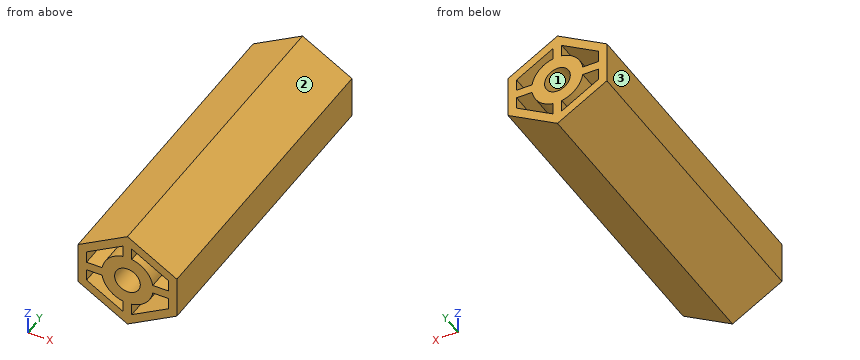
from build123d import *

# Parameters (mm, degrees)
SKETCH1_R           = 3.25
BOSS_EXTRUDE2_DEPTH = 80


with BuildPart() as part:
    # Sketch1 → Boss-Extrude2 (new body)
    with BuildSketch(Plane(origin=(0, 0, 0), x_dir=(1, 0, 0), z_dir=(0, 1, 0))):
        Polygon((-12.5, 5.283121635), (-12.5, -5.283121635), (0, -12.5), (12.5, -5.283121635), (12.5, 5.283121635), (0, 12.5), align=None)
        Circle(SKETCH1_R, mode=Mode.SUBTRACT)
        with BuildLine():
            Line((-1.08, 9.382308546), (-1.08, 6.409648976))
            ThreePointArc((-1.08, 6.409648976), (-4.596194078, 4.596194078), (-6.409648976, 1.08))
            Line((-6.409648976, 1.08), (-10.34, 1.08))
            Line((-10.34, 1.08), (-10.34, 4.036045054))
            Line((-10.34, 4.036045054), (-1.08, 9.382308546))
        make_face(mode=Mode.SUBTRACT)
        with BuildLine():
            Line((1.08, 9.382308546), (1.08, 6.409648976))
            ThreePointArc((1.08, 6.409648976), (4.596194078, 4.596194078), (6.409648976, 1.08))
            Line((6.409648976, 1.08), (10.34, 1.08))
            Line((10.34, 1.08), (10.34, 4.036045054))
            Line((10.34, 4.036045054), (1.08, 9.382308546))
        make_face(mode=Mode.SUBTRACT)
        with BuildLine():
            Line((-10.34, -1.08), (-6.409648976, -1.08))
            ThreePointArc((-6.409648976, -1.08), (-4.596194078, -4.596194078), (-1.08, -6.409648976))
            Line((-1.08, -6.409648976), (-1.08, -9.382308546))
            Line((-1.08, -9.382308546), (-10.34, -4.036045054))
            Line((-10.34, -4.036045054), (-10.34, -1.08))
        make_face(mode=Mode.SUBTRACT)
        with BuildLine():
            Line((1.08, -6.409648976), (1.08, -9.382308546))
            Line((1.08, -9.382308546), (10.34, -4.036045054))
            Line((10.34, -4.036045054), (10.34, -1.08))
            Line((10.34, -1.08), (6.409648976, -1.08))
            ThreePointArc((6.409648976, -1.08), (4.596194078, -4.596194078), (1.08, -6.409648976))
        make_face(mode=Mode.SUBTRACT)
    extrude(amount=BOSS_EXTRUDE2_DEPTH)


solid = part.part
Verification items for the finished model (mm, model axes). Face numbers are marked on the shaded views. Coordinates: 2 decimals unless noted, no trailing zeros. Loops run counter-clockwise (first coordinate to the right, second up) from the corner with the lowest first, then second, coordinate; pieces in that order, holes last. Notation, with made-up numbers: M -33.75,-37 L 18.25,-37 A21 cw 18.25,-30 Z; hole C -28,-6.5 d11. An arc over 180 degrees is marked long. One line per item, written item: value.
1. Section check B-B on x = -4. Record the cut outline in (y, z).
Answers follow:
outline: M 0,-10.19 L 80,-10.19 L 80,-7.7 L 0,-7.7 Z; M 0,-5.12 L 80,-5.12 L 80,5.12 L 0,5.12 Z; M 0,7.7 L 80,7.7 L 80,10.19 L 0,10.19 Z
2. Section check C-C on y = 24.5. Record the cut outline in (x, z).
Answers follow:
outline: M -12.5,-5.28 L 0,-12.5 L 12.5,-5.28 L 12.5,5.28 L 0,12.5 L -12.5,5.28 Z; hole M -10.34,-4.04 L -1.08,-9.38 L -1.08,-6.41 A6.5 cw -6.41,-1.08 L -10.34,-1.08 Z; hole M -10.34,1.08 L -6.41,1.08 A6.5 cw -1.08,6.41 L -1.08,9.38 L -10.34,4.04 Z; hole C 0,0 d6.5; hole M 1.08,-9.38 L 10.34,-4.04 L 10.34,-1.08 L 6.41,-1.08 A6.5 cw 1.08,-6.41 Z; hole M 1.08,6.41 A6.5 cw 6.41,1.08 L 10.34,1.08 L 10.34,4.04 L 1.08,9.38 Z
3. Section check D-D on z = -7.5. Record the cut outline in (x, y).
Answers follow:
outline: M -8.66,0 L -4.34,0 L -4.34,80 L -8.66,80 Z; M -1.08,0 L 1.08,0 L 1.08,80 L -1.08,80 Z; M 4.34,0 L 8.66,0 L 8.66,80 L 4.34,80 Z
4. Section check A-A on z = 0. Record the cut outline in (x, y), plus the area to 3 significant figures.
Answers follow:
outline: M -12.5,0 L -3.25,0 L -3.25,80 L -12.5,80 Z; M 3.25,0 L 12.5,0 L 12.5,80 L 3.25,80 Z
area: 1,480 mm^2
5. Mould release check, pull along X, two halves, no side actions. Record for the marked faces 1, 2 and 3: pulls with the +X half, pulls with the -X half, needs draft (parallel to the pull), parting line crosses it, or undercut.
Answers follow:
face 1: undercut
face 2: pulls with the +X half
face 3: pulls with the -X half
6. Material ranges on line 1 along Z through (x, y) = (-9.75, 63); line 2 along Z through (x, y) = (-7.25, 8.5); line 3 along Z through (x, y) = (0, 37.5), recorded low to high. Write a range as from..to.
Answers follow:
line 1: -6.87..-4.38, -1.08..1.08, 4.38..6.87
line 2: -8.31..-5.82, -1.08..1.08, 5.82..8.31
line 3: -12.5..-3.25, 3.25..12.5
7. Gauge pin test, flat ends, axial feed: P1, Ø2, axis at x = -9.5, y = 47, coming from the -Z side; P2, Ø0.9, axis at y = 36.5, z = -7, coming from the +X side; P3, Ø1.2, axis at x = 7.5, y = 33.5, coming from the +Z side. Record the tip position at first contact, or that the pin passes through.
Answers follow:
P1: z = -7.59
P2: x = 10.31
P3: z = 8.52
